Verification items for the finished model (mm, model axes). A direction names the side the tool comes from. Coordinates: 2 decimals unless noted, no trailing zeros. Write each loop counter-clockwise with the first axis right and the second up, starting at its lowest first coordinate (ties: lowest second). Pieces come first, ordered by that corner, then holes. Notation, with made-up numbers: (-9, 67) -> (-2, 67) arc R27 cw to (-2, 99) -> close; hole circle Ø5 at (-1, -24). An arc over 180 degrees is marked (long way). Answer in a Markdown table with one row per item.
```python
from build123d import *

# Parameters (mm, degrees)
SKETCH_1_W          = 4
SKETCH_1_H          = 4.5
EXTRUDE_1_DEPTH     = 4
SKETCH_2_W          = 0.75
SKETCH_2_H          = 0.2
CUT_EXTRUDE_1_DEPTH = 7.34428877
SKETCH_3_W          = 0.75
SKETCH_3_H          = 0.2
CUT_EXTRUDE_2_DEPTH = 4
SKETCH_4_W          = 2.5
SKETCH_4_H          = 0.2
EXTRUDE_2_DEPTH     = 0.45
SKETCH_5_W          = 2.5
SKETCH_5_H          = 0.2
EXTRUDE_3_DEPTH     = 1.707300918
SKETCH_6_W          = 3
SKETCH_6_H          = 3.3
CUT_EXTRUDE_3_DEPTH = 7.34428877
SKETCH_7_W          = 2.5
SKETCH_7_H          = 0.2
EXTRUDE_4_DEPTH     = 2.968221289
EXTRUDE_5_DEPTH     = 1
CHAMFER_1_SIZE      = 0.070710678
FILLET_1_R          = 0.05
CHAMFER_2_SIZE      = 0.2
FILLET_2_R          = 0.25


with BuildPart() as part:
    # Эскиз1 → Бобышка-Вытянуть1 (new body)
    with BuildSketch(Plane(origin=(-2, 0, 0), x_dir=(0, -1, 0), z_dir=(-1, 0, 0))):
        with Locations((0, 2.25)):
            Rectangle(SKETCH_1_W, SKETCH_1_H)
    extrude(amount=-EXTRUDE_1_DEPTH)

    # Эскиз2 → Вырез-Вытянуть1 (cut, through all)
    with BuildSketch(Plane.XZ.offset(2)):
        with Locations((-1.625, 4.4)):
            Rectangle(SKETCH_2_W, SKETCH_2_H)
    extrude(amount=-CUT_EXTRUDE_1_DEPTH, mode=Mode.SUBTRACT)

    # Эскиз3 → Вырез-Вытянуть2 (cut)
    with BuildSketch(Plane.XZ.offset(2)):
        with Locations((1.625, 4.4)):
            Rectangle(SKETCH_3_W, SKETCH_3_H)
    extrude(amount=-CUT_EXTRUDE_2_DEPTH, mode=Mode.SUBTRACT)

    # Эскиз4 → Бобышка-Вытянуть2 (add)
    with BuildSketch(Plane.XZ.offset(2)):
        with Locations((0, 4.4)):
            Rectangle(SKETCH_4_W, SKETCH_4_H)
    extrude(amount=EXTRUDE_2_DEPTH)

    # Эскиз5 → Бобышка-Вытянуть3 (add)
    with BuildSketch(Plane(origin=(0, 0, 4.3), x_dir=(-1, 0, 0), z_dir=(0, 0, -1))):
        with Locations((0, -2.35)):
            Rectangle(SKETCH_5_W, SKETCH_5_H)
    extrude(amount=EXTRUDE_3_DEPTH)

    # Эскиз6 → Вырез-Вытянуть3 (cut, through all)
    with BuildSketch(Plane.XZ.offset(2)):
        with Locations((0, 2.15)):
            Rectangle(SKETCH_6_W, SKETCH_6_H)
    extrude(amount=-CUT_EXTRUDE_3_DEPTH, mode=Mode.SUBTRACT)

    # Эскиз7 → Бобышка-Вытянуть4 (add)
    with BuildSketch(Plane(origin=(0, -2.25, 0), x_dir=(-1, 0, 0), z_dir=(0, 1, 0))):
        with Locations((0, 2.692699082)):
            Rectangle(SKETCH_7_W, SKETCH_7_H)
    extrude(amount=EXTRUDE_4_DEPTH)

    # Эскиз8 → Бобышка-Вытянуть5 (add)
    with BuildSketch(Plane.XZ):
        Polygon((-0.25, 0), (-0.25, -2.8), (0, -3.05), (0.25, -2.8), (0.25, 0), align=None)
    extrude(amount=-EXTRUDE_5_DEPTH)

    # Фаска1
    chamfer_1_edges = [part.edges().sort_by_distance(p)[0] for p in [
        (0, 0.5, -3.05),
    ]]
    chamfer(chamfer_1_edges, length=CHAMFER_1_SIZE)

    # Скругление1
    fillet_1_edges = [part.edges().sort_by_distance(p)[0] for p in [
        (0, -2.25, 4.3),
        (0, -2.25, 2.792699082),
    ]]
    fillet(fillet_1_edges, radius=FILLET_1_R)

    # Фаска2
    chamfer_2_edges = [part.edges().sort_by_distance(p)[0] for p in [
        (0, 1, -3),
        (0, 0, -3),
    ]]
    chamfer(chamfer_2_edges, length=CHAMFER_2_SIZE)

    # Скругление2
    fillet_2_edges = [part.edges().sort_by_distance(p)[0] for p in [
        (2, 0, 0),
        (-2, 0, 4.3),
        (2, 0, 4.3),
        (0, -2.45, 4.5),
        (-2, 0, 0),
        (0, -2.45, 2.592699082),
        (-1.5, 0, 0.5),
        (-1.5, 0, 3.8),
        (1.5, 0, 3.8),
        (1.5, 0, 0.5),
    ]]
    fillet(fillet_2_edges, radius=FILLET_2_R)


solid = part.part
```
1. Depth check by flat-ended pin: P1, Ø1, axis at x = 1.5, y = 0.5, coming from the -Z side; P2, Ø0.6, axis at x = 0, z = -2, coming from the -Y side. Enter the tip coordinate at first touch or a pass-through.
Geometry says:
| item | result |
|---|---|
| P1 | z = 0 |
| P2 | y = 0 |
2. Section check D-D, the plane y = 1.45. Record the boundary of the cut face in (x, z), plus the area to 3 significant figures.
Geometry says:
| item | result |
|---|---|
| outline | (-2, 0.25) arc R0.25 ccw to (-1.75, 0) -> (1.75, 0) arc R0.25 ccw to (2, 0.25) -> (2, 4.05) arc R0.25 ccw to (1.75, 4.3) -> (1.25, 4.3) -> (1.25, 4.5) -> (-1.25, 4.5) -> (-1.25, 4.3) -> (-1.75, 4.3) arc R0.25 ccw to (-2, 4.05) -> close; hole (-1.5, 0.75) arc R0.25 ccw to (-1.25, 0.5) -> (1.25, 0.5) arc R0.25 ccw to (1.5, 0.75) -> (1.5, 3.55) arc R0.25 ccw to (1.25, 3.8) -> (-1.25, 3.8) arc R0.25 ccw to (-1.5, 3.55) -> close |
| area | 7.80 mm^2 |
3. Tool access check on faces 5 (the flat face through (0, -2.25, 4)), 6 (the flat face through (0, 0, 3.8)), 7 (the flat face through (-2, 0, 2)), 8 (the flat face through (0, 0, 4.5)), 9 (the flat face through (0, -1, 2.593)). Record the directions out of +Z, -Z, +X, -X, +Y, -Y that give a thin tool (end or side, any length) a straight path to the whole face; none if there is none.
Geometry says:
| item | result |
|---|---|
| face 5 | +X, -X |
| face 6 | +Y |
| face 7 | +Z, -Z, -X, +Y, -Y |
| face 8 | +Z, +X, -X, +Y, -Y |
| face 9 | +Y, -Y |
4. Section check B-B, the plane x = 0.75. Record the boundary of the cut face in (y, z).
Geometry says:
| item | result |
|---|---|
| outline | (-2.45, 2.84) arc R0.25 ccw to (-2.2, 2.59) -> (0.72, 2.59) -> (0.72, 2.79) -> (-2.2, 2.79) arc R0.05 cw to (-2.25, 2.84) -> (-2.25, 4.25) arc R0.05 cw to (-2.2, 4.3) -> (-2, 4.3) -> (-2, 3.8) -> (2, 3.8) -> (2, 4.5) -> (-2.2, 4.5) arc R0.25 ccw to (-2.45, 4.25) -> close; (-2, 0) -> (2, 0) -> (2, 0.5) -> (-2, 0.5) -> close |
5. Mould release check, pull along X, two halves, no side actions. Record for faces 1 (the flat face through (0, 0, 0.5)), 2 (the flat face through (0.25, 0.5, -1.4)), 3 (the flat face through (1.7, 2, 2.2)), 4 (the flat face through (-0.25, 0.5, -1.4)): released by +X, released by -X, zero draft, split by the parting line, or undercut.
Geometry says:
| item | result |
|---|---|
| face 1 | undercut |
| face 2 | released by +X |
| face 3 | zero draft |
| face 4 | released by -X |
6. Thickness scan on line 1 (Z direction, x = 0.3, y = -1.2); line 2 (X direction, y = 0.9, z = 2); line 3 (Z direction, x = 0.35, y = 0.8). Record the ranges inside material, lowest first. Write a range as from..to.
Geometry says:
| item | result |
|---|---|
| line 1 | 0..0.5, 2.59..2.79, 3.8..4.5 |
| line 2 | -2..-1.5, 1.5..2 |
| line 3 | 0..0.5, 3.8..4.5 |
7. Section check A-A, the plane y = 0.4. State how many separate pieces and enclosed holes the cut face has, plus the area to 3 significant figures.
Geometry says:
| item | result |
|---|---|
| separate pieces | 2 |
| enclosed holes | 1 |
| area | 9.76 mm^2 |
8. Section check C-C, the plane z = 3.25. Record the boundary of the cut face in (x, y), plus the area to 3 significant figures.
Geometry says:
| item | result |
|---|---|
| outline | (-2, -2) -> (-1.5, -2) -> (-1.5, 2) -> (-2, 2) -> close; (-1.25, -2.45) -> (1.25, -2.45) -> (1.25, -2.25) -> (-1.25, -2.25) -> close; (1.5, -2) -> (2, -2) -> (2, 2) -> (1.5, 2) -> close |
| area | 4.50 mm^2 |
